from build123d import *

# Parameters (mm, degrees)
F0_W     = 406.4
F0_H     = 228.6
F1_DEPTH = 19.05
F2_W     = 12.7
F2_H     = 12.7
F3_DEPTH = 406.4
F4_W     = 19.05
F4_H     = 12.7
F5_DEPTH = 9.525


with BuildPart() as f1:
    # F0 (on Front) → F1 (new body)
    with BuildSketch(Plane.XZ):
        Rectangle(F0_W, F0_H)
    extrude(amount=F1_DEPTH)

    # F2 (on face) → F3 (cut, through all)
    with BuildSketch(Plane(origin=(-203.2, 0, 0), x_dir=(0, -1, 0), z_dir=(-1, 0, 0))):
        with Locations((6.35, 107.95)):
            Rectangle(F2_W, F2_H)
    extrude(amount=-F3_DEPTH, mode=Mode.SUBTRACT)

    # F4 (on face) → F5 (cut)
    with BuildSketch(Plane(origin=(0, 0, 0), x_dir=(-1, 0, 0), z_dir=(0, 1, 0))):
        with Locations((-193.675, 50.8)):
            Rectangle(F4_W, F4_H)
        with Locations((-193.675, 12.7)):
            Rectangle(F4_W, F4_H)
        with Locations((-193.675, -25.4)):
            Rectangle(F4_W, F4_H)
        with Locations((-193.675, -63.5)):
            Rectangle(F4_W, F4_H)
        with Locations((193.675, 50.8)):
            Rectangle(F4_W, F4_H)
        with Locations((193.675, 12.7)):
            Rectangle(F4_W, F4_H)
        with Locations((193.675, -25.4)):
            Rectangle(F4_W, F4_H)
        with Locations((193.675, -63.5)):
            Rectangle(F4_W, F4_H)
    extrude(amount=-F5_DEPTH, mode=Mode.SUBTRACT)


solid = f1.part
Can you work these out from the model? Positions are in its coordinate system, mm. A direction names the side the tool comes from. Give positions to 0.01 mm unless a question says otherwise; leave off trailing zeros. Write each loop counter-clockwise with the first axis right and the second up, starting at its lowest first coordinate (ties: lowest second). Pieces come first, ordered by that corner, then holes. Notation, with made-up numbers: (-24, 76.5) -> (10, 76.5) arc R16 cw to (10, 101.5) -> close; hole circle Ø8 at (55, 9.25). An arc over 180 degrees is marked (long way). Answer as a JSON object with one key per item and string values. Group by question number.
Item 1: Suppose I cut it at A-A (z = -66). Please give me the cut outline in (x, y) (3 decimals), plus the area to 3 significant figures.
Item 2: We'd pull the mould along Z, two halves only. Please class faces 4 (the face through (-203.2, -9, -2)), 5 (the face through (-3, -9, -114.3)), 6 (the face through (-194, -5, -31.75)), 7 (the face through (194, -9.525, 51)): +Z half, -Z half, draft (parallel to the pull), parting line (faces both ways), or undercut.
Item 3: I'm going to push flat-ended pins straight in: P1, Ø5, axis at x = -192, y = -3, coming from the +Z side; P2, Ø3, axis at y = -6, z = 51, coming from the +X side; P3, Ø6.5, axis at x = -19, z = 110, coming from the +Y side. Where does each tip first touch, or does it pass through?
Item 4: For faces 1 (the face through (-3, -12.7, 108)), 2 (the face through (-194, -5, 57.15)), 3 (the face through (184.15, -5, 51)), which set-ups out of +Z, -Z, +X, -X, +Y, -Y let a thin tool reach every point of the face, with its end or its side?
Item 5: Please list where these lines run through material, in increasing order: line 1 (Z direction, x = 106, y = -7); line 2 (X direction, y = -3.75, z = -65). Write a range as [from, to].
Item 6: Suppose I cut it at B-B (x = -21.5). Please give me the cut outline in (y, z).
Findings:
{
 "1": {"outline": "(-203.2, -19.05) -> (203.2, -19.05) -> (203.2, -9.525) -> (184.15, -9.525) -> (184.15, 0) -> (-184.15, 0) -> (-184.15, -9.525) -> (-203.2, -9.525) -> close", "area": "7,380 mm²"},
 "2": {"face 4": "draft", "face 5": "-Z half", "face 6": "undercut", "face 7": "undercut"},
 "3": {"P1": "stops at z = 101.6", "P2": "stops at x = 184.15", "P3": "stops at y = -12.7"},
 "4": {"face 1": "+Z, +X, -X, +Y", "face 2": "-X, +Y", "face 3": "+X, +Y"},
 "5": {"line 1": "z = [-114.3, 101.6]", "line 2": "x = [-184.15, 184.15]"},
 "6": {"outline": "(-19.05, -114.3) -> (0, -114.3) -> (0, 101.6) -> (-12.7, 101.6) -> (-12.7, 114.3) -> (-19.05, 114.3) -> close"}
}
